```python
from build123d import *

# Parameters (mm, degrees)
F2_R     = 1.5875
F3_R     = 3.175
F4_DEPTH = 1.5875


with BuildPart() as f1:
    # F0 (on Right) → F1 (revolve)
    with BuildSketch(Plane.YZ):
        with BuildLine():
            Line((-144.4625, 12.7), (-149.225, 12.7))
            Line((-149.225, 12.7), (-149.225, 0))
            Line((-149.225, 0), (-136.525, 0))
            Line((-136.525, 0), (152.4, 0))
            Line((152.4, 0), (152.4, 1.5875))
            Line((152.4, 1.5875), (-136.525, 1.5875))
            Line((-136.525, 1.5875), (-136.525, 12.7))
            Line((-136.525, 12.7), (-141.2875, 12.7))
            ThreePointArc((-141.2875, 12.7), (-142.875, 11.1125), (-144.4625, 12.7))
        make_face()
    revolve(axis=Axis((0, 7.9375, 0), (0, 1, 0)))

    # F2
    f2_edges = [f1.edges().sort_by_distance(p)[0] for p in [
        (0, -136.525, -12.7),
        (0, -149.225, -12.7),
    ]]
    fillet(f2_edges, radius=F2_R)

    # F3 (on face) → F4 (join)
    with BuildSketch(Plane(origin=(0, 152.4, 0), x_dir=(-1, 0, 0), z_dir=(0, 1, 0))):
        Circle(F3_R)
    extrude(amount=F4_DEPTH)


solid = f1.part
```
Could you check a few things on this model? Use its own coordinates, in mm. A direction names the side the tool comes from. Give positions to 0.01 mm unless a question says otherwise; leave off trailing zeros. Loops run counter-clockwise (first coordinate to the right, second up) from the corner with the lowest first, then second, coordinate; pieces in that order, holes last. Notation, with made-up numbers: (18, 12.25) -> (53, 12.25) arc R23 ccw to (53, 30.25) -> close; hole circle Ø9 at (55.25, 42.25). An arc over 180 degrees is marked (long way). Put each result on its own line as item: value.
(1) Please list where these lines run through material, in increasing order: probe 1 along Y at (x, z) = (-5.5, 6.5) (3 decimals); probe 2 along X at (y, z) = (91, 0); probe 3 along Y at (x, z) = (-4.5, -10.5). Write a range as [from, to].
Computed:
probe 1: [-149.225, -136.525]
probe 2: [-1.59, 1.59]
probe 3: [-149.19, -143.82], [-141.93, -136.56]
(2) I'm going to push flat-ended pins straight in: pin 1 Ø8 at (x, y) = (-3, -100) entering from -Z; pin 2 Ø5 at (x, y) = (-2.5, -81.5) entering from +Z; pin 3 Ø8 at (y, z) = (36.5, -2) entering from -X. Where does each tip first touch, or does it pass through?
Computed:
pin 1: z = -1.59
pin 2: z = 1.59
pin 3: x = -1.59
(3) Thinking about a two-plate mould opening in Y: for faces 3 (the face through (0, -149.225, 0)), 4 (the face through (-12.4, -139.72, -2.75)), 5 (the face through (-1.4, 152.4, -1.4)), which applies, pulls with the +Y half, pulls with the -Y half, needs draft (parallel to the pull), parting line crosses it, or undercut?
Computed:
face 3: pulls with the -Y half
face 4: needs draft
face 5: undercut
(4) Imagine slicing it at A-A on y = -80.5. Write out the boundary of the cut face in (x, z) (1 decimal).
Computed:
outline: circle Ø3.2 at (0, 0)
(5) For faces 1 (the face through (0, 153.988, 0)), 2 (the face through (0.69, 153.18, -3.1)), which set-ups out of +Z, -Z, +X, -X, +Y, -Y let a thin tool reach every point of the face, with its end or its side?
Computed:
face 1: +Z, -Z, +X, -X, +Y
face 2: +Y
